The model under review builds one solid part; all positions refer to its coordinate system, in mm. Coordinates: 2 decimals unless noted, no trailing zeros. Order: outer loops, then holes, each group sorted by start corner. A loop starts at its lowest first (then second) coordinate and runs counter-clockwise, first axis right, second up. Notation, with made-up numbers: M -1,-7 L 55,-7 A34 ccw 55,24 Z; hole C 68.5,-21.5 d7. An arc over 180 degrees is marked long. Answer in a Markdown table with one row per item.
from build123d import *

# Parameters (mm, degrees)
BOSS_EXTRUDE1_DEPTH                  = 342.9
BOSS_EXTRUDE1_DEPTH_BACK             = 342.9
SKETCH3_W                            = 38.1
SKETCH3_H                            = 25.4
SKETCH3_W_2                          = 31.75
SKETCH3_H_2                          = 19.05
F_1_4_0_25_DIAMETER_HOLE2_AT_2_COUNT = 2
F_1_4_0_25_DIAMETER_HOLE2_AT_2_PITCH = 25.4
F_1_4_0_25_DIAMETER_HOLE2_AT_3_COUNT = 2
F_1_4_0_25_DIAMETER_HOLE2_AT_3_PITCH = 661.111799988
F_1_4_0_25_DIAMETER_HOLE2_AT_4_COUNT = 2
F_1_4_0_25_DIAMETER_HOLE2_AT_4_PITCH = 50.8
F_1_4_0_25_DIAMETER_HOLE2_AT_5_COUNT = 2
F_1_4_0_25_DIAMETER_HOLE2_AT_5_PITCH = 635.711799988
F_1_4_0_25_DIAMETER_HOLE3_D          = 6.35
F_5_32_0_15625_DIAMETER_HOLE1_D      = 3.96875
F_10_CLEARANCE_HOLE1_D               = 5.1054


with BuildPart() as part:
    # Sketch3 → Boss-Extrude1 (new, two sides: drawn at the far end of the back side and taken through both)
    with BuildSketch(Plane.XY.offset(-BOSS_EXTRUDE1_DEPTH_BACK)):
        Rectangle(SKETCH3_W, SKETCH3_H)
        Rectangle(SKETCH3_W_2, SKETCH3_H_2, mode=Mode.SUBTRACT)
    extrude(amount=BOSS_EXTRUDE1_DEPTH + BOSS_EXTRUDE1_DEPTH_BACK)

    # Sketch8 → 1/4 (0.25) Diameter Hole2 (revolve, cut)
    with BuildSketch(Plane(origin=(-19.05, 0, -330.2), x_dir=(0, 0, 1), z_dir=(0, 1, 0))):
        Polygon((0, 0), (0, 38.1), (3.9624, 38.1), (3.175, 37.194199916), (3.175, 0), align=None)
    f_1_4_0_25_diameter_hole2 = revolve(axis=Axis((-25.4, 0, -330.2), (1, 0, 0)), mode=Mode.SUBTRACT)

    # 1/4 (0.25) Diameter Hole2 at 2: 1/4 (0.25) Diameter Hole2 ×2
    with Locations(*[(0, 0, i * F_1_4_0_25_DIAMETER_HOLE2_AT_2_PITCH) for i in range(1, F_1_4_0_25_DIAMETER_HOLE2_AT_2_COUNT)]):
        add(f_1_4_0_25_diameter_hole2, mode=Mode.SUBTRACT)

    # 1/4 (0.25) Diameter Hole2 at 3: 1/4 (0.25) Diameter Hole2 ×2
    with Locations(*[(0, 0, i * F_1_4_0_25_DIAMETER_HOLE2_AT_3_PITCH) for i in range(1, F_1_4_0_25_DIAMETER_HOLE2_AT_3_COUNT)]):
        add(f_1_4_0_25_diameter_hole2, mode=Mode.SUBTRACT)

    # 1/4 (0.25) Diameter Hole2 at 4: 1/4 (0.25) Diameter Hole2 ×2
    with Locations(*[(0, 0, i * F_1_4_0_25_DIAMETER_HOLE2_AT_4_PITCH) for i in range(1, F_1_4_0_25_DIAMETER_HOLE2_AT_4_COUNT)]):
        add(f_1_4_0_25_diameter_hole2, mode=Mode.SUBTRACT)

    # 1/4 (0.25) Diameter Hole2 at 5: 1/4 (0.25) Diameter Hole2 ×2
    with Locations(*[(0, 0, i * F_1_4_0_25_DIAMETER_HOLE2_AT_5_PITCH) for i in range(1, F_1_4_0_25_DIAMETER_HOLE2_AT_5_COUNT)]):
        add(f_1_4_0_25_diameter_hole2, mode=Mode.SUBTRACT)

    # 1/4 (0.25) Diameter Hole3 (through all)
    with Locations(Plane(origin=(19.05, 0, 0), x_dir=(0, 0, -1), z_dir=(1, 0, 0))):
        with Locations((-280.111799988, 0), (-254.711799988, 0), (-229.311799988, 0), (254, 0), (228.6, 0), (203.2, 0)):
            Hole(F_1_4_0_25_DIAMETER_HOLE3_D / 2)

    # 5/32 (0.15625) Diameter Hole1 (through all)
    with Locations(Plane(origin=(19.05, 0, 0), x_dir=(0, 0, -1), z_dir=(1, 0, 0))):
        with Locations((152.4, 0), (-178.511799988, 0)):
            Hole(F_5_32_0_15625_DIAMETER_HOLE1_D / 2)

    # #10 Clearance Hole1 (through all)
    with Locations(Plane(origin=(19.05, 0, 0), x_dir=(0, 0, -1), z_dir=(1, 0, 0))):
        with Locations((-128.943395188, 0.344528206), (-103.543395188, 0.344528206), (77.4315952, -0.000599988), (102.8315952, -0.000599988)):
            Hole(F_10_CLEARANCE_HOLE1_D / 2)


solid = part.part
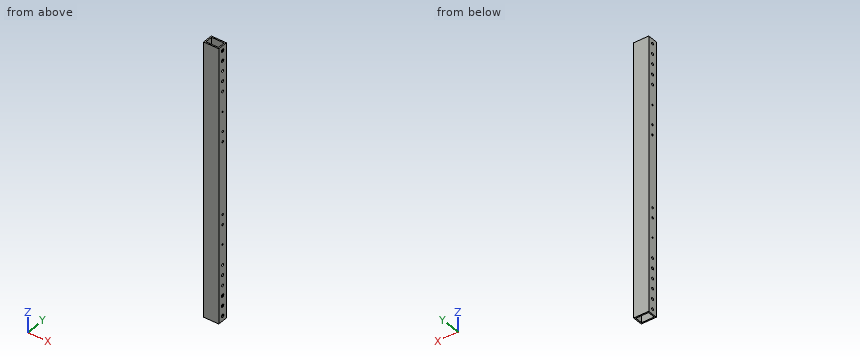
(1) Insertion check: P1, Ø8, axis at y = 0.34, z = 128.94, coming from the +X side; P2, Ø2, axis at x = -13, y = -4, coming from the -Z side. Each pin has a flat end and moves straight along its axis. Give the tip position at first contact, or say it passes through.
Report:
| item | result |
|---|---|
| P1 | x = 19.05 |
| P2 | through |
(2) To check wall thickness, follow line 1 (Y direction, x = -8, z = 132.5) (3 decimals); line 2 (X direction, y = -4.5, z = 177.5) (3 decimals); line 3 (Y direction, x = -18, z = -203.2) (3 decimals). State the ranges of each line that lie inside material, in increasing order. Write a range as [from, to].
Report:
| item | result |
|---|---|
| line 1 | [-12.7, -9.525], [9.525, 12.7] |
| line 2 | [-19.05, -15.875], [15.875, 19.05] |
| line 3 | [-12.7, -3.175], [3.175, 12.7] |
(3) Take a section at A-A (x = -2.5). Write out the cut boundary in (y, z) (3 decimals).
Report:
| item | result |
|---|---|
| outline | M -12.7,-342.9 L -9.525,-342.9 L -9.525,342.9 L -12.7,342.9 Z; M 9.525,-342.9 L 12.7,-342.9 L 12.7,342.9 L 9.525,342.9 Z |
(4) Take a section at B-B (z = 21.5). Write out the cut boundary in (x, y) (3 decimals), then the cut area to 3 significant figures.
Report:
| item | result |
|---|---|
| outline | M -19.05,-12.7 L 19.05,-12.7 L 19.05,12.7 L -19.05,12.7 Z; hole M -15.875,-9.525 L 15.875,-9.525 L 15.875,9.525 L -15.875,9.525 Z |
| area | 363 mm^2 |
